Input: part model. Units: mm. Frame: model coordinates. Give positions to 0.01 mm unless a question says otherwise; leave off trailing zeros. Use CSV: the item, a comma, the result in double quotes. Start each with the question number.
Q1. Pin query (flat end, axial travel): pin 1 (1 mm diameter, centred on x = 4, z = -93, fed in from +Y); pin 2 (2 mm diameter, centred on x = 7, y = 41, fed in from -Z). Return the tip coordinate at first contact, or that it passes through.
Q2. Material intervals for line 1 along Y through (x, z) = (5.5, 0); line 2 along Z through (x, y) = (4.5, 3); line 3 along Y through (x, z) = (6.75, -93.5), sorted ascending.
Q3. Section A-A, the plane x = 1.75. State how many separate pieces and enclosed holes the cut face has, plus the area to 3 significant figures.
Q4. Pull-direction query (Z, two-part tool) for faces 1 (the cylindrical face through (4.06, -4.56, 124.7)), 2 (the cylindrical face through (3.948, 154.672, 20.308)), 3 (the flat face through (0, -32, 2)); classes: released by +Z, released by -Z, zero draft, split by the parting line, or undercut.
from build123d import *

# Parameters (mm, degrees)
SKETCH_1_R               = 156
EXTRUDE_1_DEPTH          = 8
SKETCH_2_R               = 30
CUT_EXTRUDE_1_DEPTH      = 10
SKETCH_3_R               = 35
CUT_EXTRUDE_2_DEPTH      = 10
PATTERN_CIRCULAR_1_COUNT = 4
SKETCH_4_R               = 6
CUT_EXTRUDE_3_DEPTH      = 10
PATTERN_CIRCULAR_2_COUNT = 4
SKETCH_6_R               = 2.5
CUT_EXTRUDE_5_DEPTH      = 10
PATTERN_CIRCULAR_4_COUNT = 4
FILLET_1_R               = 0.3


with BuildPart() as part:
    # 草图1 → 凸台-拉伸1 (new body)
    with BuildSketch(Plane(origin=(0, 0, 0), x_dir=(0, 0, -1), z_dir=(1, 0, 0))):
        Circle(SKETCH_1_R)
    extrude(amount=EXTRUDE_1_DEPTH)

    # 草图2 → 切除-拉伸1 (cut)
    with BuildSketch(Plane(origin=(8, 0, 0), x_dir=(0, 0, -1), z_dir=(1, 0, 0))):
        Circle(SKETCH_2_R)
    extrude(amount=-CUT_EXTRUDE_1_DEPTH, mode=Mode.SUBTRACT)

    # 草图3 → 切除-拉伸2 (cut)
    with BuildSketch(Plane(origin=(8, 0, 0), x_dir=(0, 0, -1), z_dir=(1, 0, 0))):
        with Locations((0, 90)):
            Circle(SKETCH_3_R)
    cut_extrude_2 = extrude(amount=-CUT_EXTRUDE_2_DEPTH, mode=Mode.SUBTRACT)

    # 阵列(圆周)1: 切除-拉伸2 ×4 about axis
    pattern_circular_1_axis = Axis((0, 0, 0), (1, 0, 0))
    for i in range(1, PATTERN_CIRCULAR_1_COUNT):
        add(cut_extrude_2.rotate(pattern_circular_1_axis, i * 360 / PATTERN_CIRCULAR_1_COUNT), mode=Mode.SUBTRACT)

    # 草图4 → 切除-拉伸3 (cut)
    with BuildSketch(Plane(origin=(8, 0, 0), x_dir=(0, 0, -1), z_dir=(1, 0, 0))):
        with Locations((91.923881554, 91.923881554)):
            Circle(SKETCH_4_R)
    cut_extrude_3 = extrude(amount=-CUT_EXTRUDE_3_DEPTH, mode=Mode.SUBTRACT)

    # 阵列(圆周)2: 切除-拉伸3 ×4 about axis
    pattern_circular_2_axis = Axis((0, 0, 0), (1, 0, 0))
    for i in range(1, PATTERN_CIRCULAR_2_COUNT):
        add(cut_extrude_3.rotate(pattern_circular_2_axis, i * 360 / PATTERN_CIRCULAR_2_COUNT), mode=Mode.SUBTRACT)

    # 草图6 → 切除-拉伸5 (cut)
    with BuildSketch(Plane(origin=(8, 0, 0), x_dir=(0, 0, -1), z_dir=(1, 0, 0))):
        with Locations((0, 35)):
            Circle(SKETCH_6_R)
    cut_extrude_5 = extrude(amount=-CUT_EXTRUDE_5_DEPTH, mode=Mode.SUBTRACT)

    # 阵列(圆周)4: 切除-拉伸5 ×4 about axis
    pattern_circular_4_axis = Axis((0, 0, 0), (1, 0, 0))
    for i in range(1, PATTERN_CIRCULAR_4_COUNT):
        add(cut_extrude_5.rotate(pattern_circular_4_axis, i * 360 / PATTERN_CIRCULAR_4_COUNT), mode=Mode.SUBTRACT)

    # 圆角1
    fillet_1_edges = [part.edges().sort_by_distance(p)[0] for p in [
        (0, 0, 156),
        (8, 0, 156),
    ]]
    fillet(fillet_1_edges, radius=FILLET_1_R)


solid = part.part
A:
1,pin 1,"y = 125.62"
1,pin 2,"z = -150.78"
2,line 1,"-156 to -125, -55 to -37.5, -32.5 to -30, 30 to 32.5, 37.5 to 55, 125 to 156"
2,line 2,"-155.97 to -124.87, -55.13 to -29.85, 29.85 to 55.13, 124.87 to 155.97"
2,line 3,"-124.87 to -97.71, -86.13 to -34.82, 34.82 to 86.13, 97.71 to 124.87"
3,separate pieces,"1"
3,enclosed holes,"13"
3,area,"57,700 mm^2"
4,face 1,"undercut"
4,face 2,"split by the parting line"
4,face 3,"zero draft"
